Part print with two shaded views. Sizes in mm from the minimum x, y, z corner. A direction names the side the tool comes from. Give positions to 0.01 mm unless a question says otherwise; leave off trailing zeros. Write each loop counter-clockwise with the first axis right and the second up, starting at its lowest first coordinate (ties: lowest second). Pieces come first, ordered by that corner, then holes.
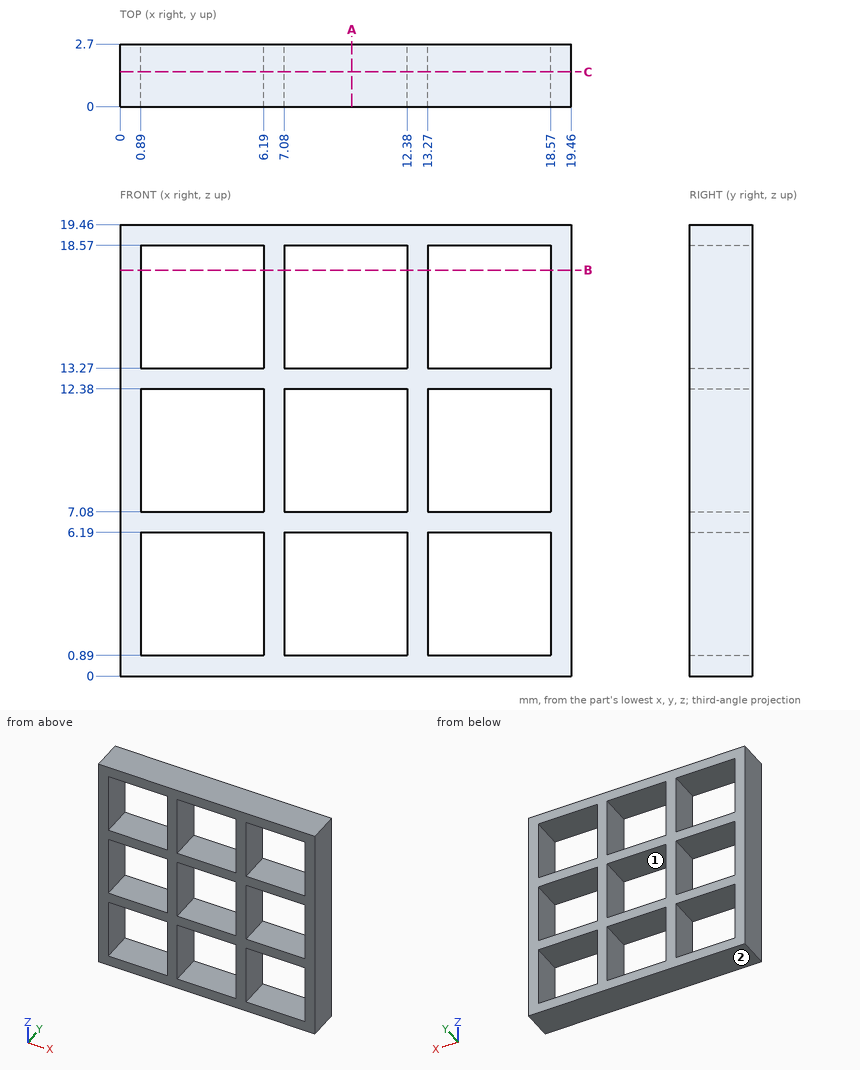
1) 3-axis set-ups, long thin cutter, end or side, ignore diameter. For the marked faces 1 and 2: which of +Z, -Z, +X, -X, +Y, -Y reach the whole face in a straight line?
Check result:
face 1: +Y, -Y
face 2: -Z, +X, -X, +Y, -Y
2) Saw through at A-A (x = 10). Write the cut outline in (y, z).
Check result:
outline: (0, 0) - (2.7, 0) - (2.7, 0.89) - (0, 0.89) - close; (0, 6.19) - (2.7, 6.19) - (2.7, 7.08) - (0, 7.08) - close; (0, 12.38) - (2.7, 12.38) - (2.7, 13.27) - (0, 13.27) - close; (0, 18.57) - (2.7, 18.57) - (2.7, 19.46) - (0, 19.46) - close
3) Drill centre line: L1, parallel to Z at x = 7.75, y = 2.35. Where is it in solid material? Low to high.
Check result:
L1: z = 0 to 0.89, 6.19 to 7.08, 12.38 to 13.27, 18.57 to 19.46
4) Saw through at C-C (y = 1.5). State how many separate pieces and enclosed holes the cut face has, and give its area (3 significant figures).
Check result:
separate pieces: 1
enclosed holes: 9
area: 126 mm2
5) Saw through at B-B (z = 17.5). Write the cut outline in (x, y), and give its area (3 significant figures).
Check result:
outline: (0, 0) - (0.89, 0) - (0.89, 2.7) - (0, 2.7) - close; (6.19, 0) - (7.08, 0) - (7.08, 2.7) - (6.19, 2.7) - close; (12.38, 0) - (13.27, 0) - (13.27, 2.7) - (12.38, 2.7) - close; (18.57, 0) - (19.46, 0) - (19.46, 2.7) - (18.57, 2.7) - close
area: 9.61 mm2
